Read the model definition and answer for the solid it produces. Units are mm, in the model's axes. A direction names the side the tool comes from. Round coordinates to 2 decimals unless told otherwise and drop trailing zeros. Order: outer loops, then holes, each group sorted by start corner. A loop starts at its lowest first (then second) coordinate and runs counter-clockwise, first axis right, second up. Notation, with made-up numbers: (18, -36) - (29, -36) arc R20 ccw to (29, -28) - close; hole circle Ø3 at (39.5, -10.75). An arc over 180 degrees is marked (long way). Answer as a JSON object with one key per item and string values. Group by question number.
Q1. Consider line 1 (X direction, y = 37, z = 2.5) (3 decimals); line 2 (Z direction, x = 71.5, y = 25); line 3 (X direction, y = 25, z = 11.25). Determine where each line is inside the solid, lowest interval first.
Q2. A cutting plane is placed at C-C on z = 14.5. Determine the outline of the cut face in (x, y) (3 decimals).
Q3. A cutting plane is placed at A-A on y = 6.5. Determine the outline of the cut face in (x, z) (3 decimals), and give its area (3 significant figures).
Q4. Given pin 1 Ø1.5 at (x, y) = (66, 19.5) entering from -Z; pin 2 Ø8 at (y, z) = (25.4, 9.525) entering from -X; pin 3 Ø5 at (x, z) = (19.5, 12.5) entering from +Y; pin 4 Ø7.5 at (x, z) = (56.5, 12) entering from -Y, each flat-ended and moving along its own axis, determine where each tip first touches the part or whether it passes through.
Q5. A tool of negligible diameter and unlimited length cuts with its end or side. For faces 4 (the flat face through (50.8, 19, 9)), 5 (the flat face through (50, 50.8, 9)), 6 (the cylindrical face through (8.049, 31.892, 10.377)), 7 (the flat face through (15.875, 36, 9)), from which of +Z, -Z, +X, -X, +Y, -Y can it reach the whole face along a straight path? Write none if from no direction.
Q6. A cutting plane is placed at B-B on y = 25.4. Determine the outline of the cut face in (x, z) (3 decimals), and give its area (3 significant figures).
Q7. A cutting plane is placed at D-D on x = 8.5. Determine the outline of the cut face in (y, z) (3 decimals), and give its area (3 significant figures).
Q8. The mould has two halves that part along Y. Classify faces 1 (the cylindrical face through (68.151, 31.892, 8.673)), 2 (the flat face through (56, 38.1, 9)), 3 (the flat face through (39, 26, 19.05)): pulls with the +Y half, pulls with the -Y half, needs draft (parallel to the pull), parting line crosses it, or undercut.
```python
from build123d import *

# Parameters (mm, degrees)
BOSS_EXTRUDE1_DEPTH         = 19.05
F_1_2_CLEARANCE_HOLE1_D     = 13.09624
F_1_2_CLEARANCE_HOLE1_DEPTH = 15.875
F_1_2_CLEARANCE_HOLE2_D     = 13.09624
F_1_2_CLEARANCE_HOLE2_DEPTH = 15.875


with BuildPart() as part:
    # Sketch1 → Boss-Extrude1 (new body)
    with BuildSketch(Plane.XY):
        Polygon((0, 0), (0, 50.8), (15.875, 50.8), (15.875, 12.7), (25.4, 12.7), (25.4, 50.8), (76.2, 50.8), (76.2, 0), (60.325, 0), (60.325, 38.1), (50.8, 38.1), (50.8, 0), align=None)
    extrude(amount=BOSS_EXTRUDE1_DEPTH)

    # 1/2 Clearance Hole1
    with Locations(Plane.ZY):
        with Locations((9.525, 25.4)):
            Hole(F_1_2_CLEARANCE_HOLE1_D / 2, depth=F_1_2_CLEARANCE_HOLE1_DEPTH)

    # 1/2 Clearance Hole2
    with Locations(Plane(origin=(76.2, 0, 0), x_dir=(0, 0, -1), z_dir=(1, 0, 0))):
        with Locations((-9.525, 25.4)):
            Hole(F_1_2_CLEARANCE_HOLE2_D / 2, depth=F_1_2_CLEARANCE_HOLE2_DEPTH)


solid = part.part
```
Result set:
{
 "1": {"line 1": "x = 0 to 15.875, 25.4 to 50.8, 60.325 to 76.2", "line 2": "z = 0 to 2.99, 16.06 to 19.05", "line 3": "x = 25.4 to 50.8"},
 "2": {"outline": "(0, 0) - (50.8, 0) - (50.8, 38.1) - (60.325, 38.1) - (60.325, 29.658) - (76.2, 29.658) - (76.2, 50.8) - (25.4, 50.8) - (25.4, 12.7) - (15.875, 12.7) - (15.875, 21.142) - (0, 21.142) - close; (0, 29.658) - (15.875, 29.658) - (15.875, 50.8) - (0, 50.8) - close; (60.325, 0) - (76.2, 0) - (76.2, 21.142) - (60.325, 21.142) - close"},
 "3": {"outline": "(0, 0) - (50.8, 0) - (50.8, 19.05) - (0, 19.05) - close; (60.325, 0) - (76.2, 0) - (76.2, 19.05) - (60.325, 19.05) - close", "area": "1,270 mm²"},
 "4": {"pin 1": "stops at z = 0", "pin 2": "stops at x = 25.4", "pin 3": "stops at y = 12.7", "pin 4": "stops at y = 38.1"},
 "5": {"face 4": "+Z, -Z, -Y", "face 5": "+Z, -Z, +X, -X, +Y", "face 6": "-X", "face 7": "+Z, -Z, +Y"},
 "6": {"outline": "(0, 0) - (15.875, 0) - (15.875, 2.977) - (0, 2.977) - close; (0, 16.073) - (15.875, 16.073) - (15.875, 19.05) - (0, 19.05) - close; (25.4, 0) - (50.8, 0) - (50.8, 19.05) - (25.4, 19.05) - close; (60.325, 0) - (76.2, 0) - (76.2, 2.977) - (60.325, 2.977) - close; (60.325, 16.073) - (76.2, 16.073) - (76.2, 19.05) - (60.325, 19.05) - close", "area": "673 mm²"},
 "7": {"outline": "(0, 0) - (50.8, 0) - (50.8, 19.05) - (0, 19.05) - close; hole circle Ø13.096 at (25.4, 9.525)", "area": "833 mm²"},
 "8": {"face 1": "undercut", "face 2": "pulls with the -Y half", "face 3": "needs draft"}
}
